from build123d import *

# Parameters (mm, degrees)
SKETCH1_R           = 2.1
BOSS_EXTRUDE1_DEPTH = 15
CUT_EXTRUDE3_START  = -14.483913
SKETCH2_W           = 24
SKETCH2_H           = 24
CUT_EXTRUDE3_DEPTH  = 14.483913
CUT_EXTRUDE4_REACH  = 26
SKETCH3_R           = 1.7


with BuildPart() as part:
    # Sketch1 → Boss-Extrude1 (new body, symmetric)
    with BuildSketch(Plane(origin=(0, 0, 0), x_dir=(0, 0, -1), z_dir=(1, 0, 0))):
        Polygon((0, 0), (24, 0), (24, 3), (14.483913001, 3), (8, 8.960936807), (8, 24), (0, 24), align=None)
        with Locations((4, 6)):
            Circle(SKETCH1_R, mode=Mode.SUBTRACT)
        with Locations((4, 18)):
            Circle(SKETCH1_R, mode=Mode.SUBTRACT)
    extrude(amount=BOSS_EXTRUDE1_DEPTH, both=True)

    # Sketch2 → Cut-Extrude3 (cut)
    with BuildSketch(Plane.XY.offset(CUT_EXTRUDE3_START)):
        with Locations((0, 12)):
            Rectangle(SKETCH2_W, SKETCH2_H)
    extrude(amount=CUT_EXTRUDE3_DEPTH, mode=Mode.SUBTRACT)

    # Sketch3 → Cut-Extrude4 (cut, up to next)
    with BuildSketch(Plane(origin=(0, 0, 0), x_dir=(1, 0, 0), z_dir=(0, 1, 0)), mode=Mode.PRIVATE) as cut_extrude4_sk1:
        with Locations((-10, 19.241956501)):
            Circle(SKETCH3_R)
    cut_extrude4_tool1 = extrude(cut_extrude4_sk1.sketch, amount=CUT_EXTRUDE4_REACH, mode=Mode.PRIVATE) & part.part
    add(cut_extrude4_tool1.solids().sort_by_distance((-10, 0, -19.241957))[0], mode=Mode.SUBTRACT)
    # Sketch3 → Cut-Extrude4 (cut, up to next)
    with BuildSketch(Plane(origin=(0, 0, 0), x_dir=(1, 0, 0), z_dir=(0, 1, 0)), mode=Mode.PRIVATE) as cut_extrude4_sk2:
        with Locations((10, 19.241956501)):
            Circle(SKETCH3_R)
    cut_extrude4_tool2 = extrude(cut_extrude4_sk2.sketch, amount=CUT_EXTRUDE4_REACH, mode=Mode.PRIVATE) & part.part
    add(cut_extrude4_tool2.solids().sort_by_distance((10, 0, -19.241957))[0], mode=Mode.SUBTRACT)


solid = part.part
The model under review builds one solid part; all positions refer to its coordinate system, in mm. A direction names the side the tool comes from. Coordinates: 2 decimals unless noted, no trailing zeros. Write each loop counter-clockwise with the first axis right and the second up, starting at its lowest first coordinate (ties: lowest second). Pieces come first, ordered by that corner, then holes. Notation, with made-up numbers: (-11.75, -17.75) -> (38.25, -17.75) arc R15 cw to (38.25, -6.75) -> close; hole circle Ø1 at (38, -20.5). An arc over 180 degrees is marked (long way). Answer in a Markdown table with one row per item.
1. We need section C-C, the plane y = 18. State the section outline as (x, z) points.
Answers below:
| item | result |
|---|---|
| outline | (-15, -8) -> (-12, -8) -> (-12, -6.1) -> (-15, -6.1) -> close; (-15, -1.9) -> (-12, -1.9) -> (-12, 0) -> (-15, 0) -> close; (12, -8) -> (15, -8) -> (15, -6.1) -> (12, -6.1) -> close; (12, -1.9) -> (15, -1.9) -> (15, 0) -> (12, 0) -> close |
2. We need section B-B, the plane y = 14.5. State the section outline as (x, z) points, and give its area (3 significant figures).
Answers below:
| item | result |
|---|---|
| outline | (-15, -8) -> (-12, -8) -> (-12, 0) -> (-15, 0) -> close; (12, -8) -> (15, -8) -> (15, 0) -> (12, 0) -> close |
| area | 48.0 mm^2 |
3. We need section D-D, the plane x = 10. State the section outline as (y, z) points, and give its area (3 significant figures).
Answers below:
| item | result |
|---|---|
| outline | (0, -24) -> (3, -24) -> (3, -20.94) -> (0, -20.94) -> close; (0, -17.54) -> (3, -17.54) -> (3, -14.48) -> (0, -14.48) -> close |
| area | 18.3 mm^2 |
4. Draft analysis for pull direction Z (two halves, no side actions). For faces 4 (the flat face through (-13, 12, 0)), 5 (the cylindrical face through (-9.09, 1.48, -20.68)), 6 (the flat face through (15, 10, -6)), state which applies: +Z half, -Z half, draft (parallel to the pull), parting line (faces both ways), or undercut.
Answers below:
| item | result |
|---|---|
| face 4 | +Z half |
| face 5 | undercut |
| face 6 | draft |
5. We need section A-A, the plane z = -4. State the section outline as (x, y) points, and give its area (3 significant figures).
Answers below:
| item | result |
|---|---|
| outline | (-15, 0) -> (-12, 0) -> (-12, 3.9) -> (-15, 3.9) -> close; (-15, 8.1) -> (-12, 8.1) -> (-12, 15.9) -> (-15, 15.9) -> close; (-15, 20.1) -> (-12, 20.1) -> (-12, 24) -> (-15, 24) -> close; (12, 0) -> (15, 0) -> (15, 3.9) -> (12, 3.9) -> close; (12, 8.1) -> (15, 8.1) -> (15, 15.9) -> (12, 15.9) -> close; (12, 20.1) -> (15, 20.1) -> (15, 24) -> (12, 24) -> close |
| area | 93.6 mm^2 |
6. Clearance check with flat-ended pins moving along their axes: pin 1 Ø10 at (x, y) = (3, 20) entering from -Z; pin 2 Ø0.9 at (x, y) = (13, 17) entering from -Z; pin 3 Ø0.9 at (x, y) = (4, 1) entering from +Z; pin 4 Ø2 at (x, z) = (5.5, -17) entering from +Y. State where each tip first meets the part, or that it passes through.
Answers below:
| item | result |
|---|---|
| pin 1 | passes through |
| pin 2 | stops at z = -8 |
| pin 3 | stops at z = -14.48 |
| pin 4 | stops at y = 3 |
7. Wall thickness on probe 1 along Z at (x, y) = (10, 1.7); probe 2 along X at (y, z) = (1.5, -4.75); probe 3 along Y at (x, z) = (-13.05, -4): over which ranges is each line inside the solid? List them lowest first. Write a range as [from, to].
Answers below:
| item | result |
|---|---|
| probe 1 | z = [-24, -20.94], [-17.54, -14.48] |
| probe 2 | x = [-15, -12], [12, 15] |
| probe 3 | y = [0, 3.9], [8.1, 15.9], [20.1, 24] |
8. For faces 1 (the cylindrical face through (13.48, 7.77, -5.13)), 2 (the flat face through (12, 9, -6)), 3 (the flat face through (-13, 16, -8)), list the 3-axis set-ups (+Z, -Z, +X, -X, +Y, -Y) from which the entire face can be reached by the end or side of a thin tool; tool diameter is ignored.
Answers below:
| item | result |
|---|---|
| face 1 | +X, -X |
| face 2 | +Z, +Y, -Y |
| face 3 | -Z, +X, -X, +Y |
